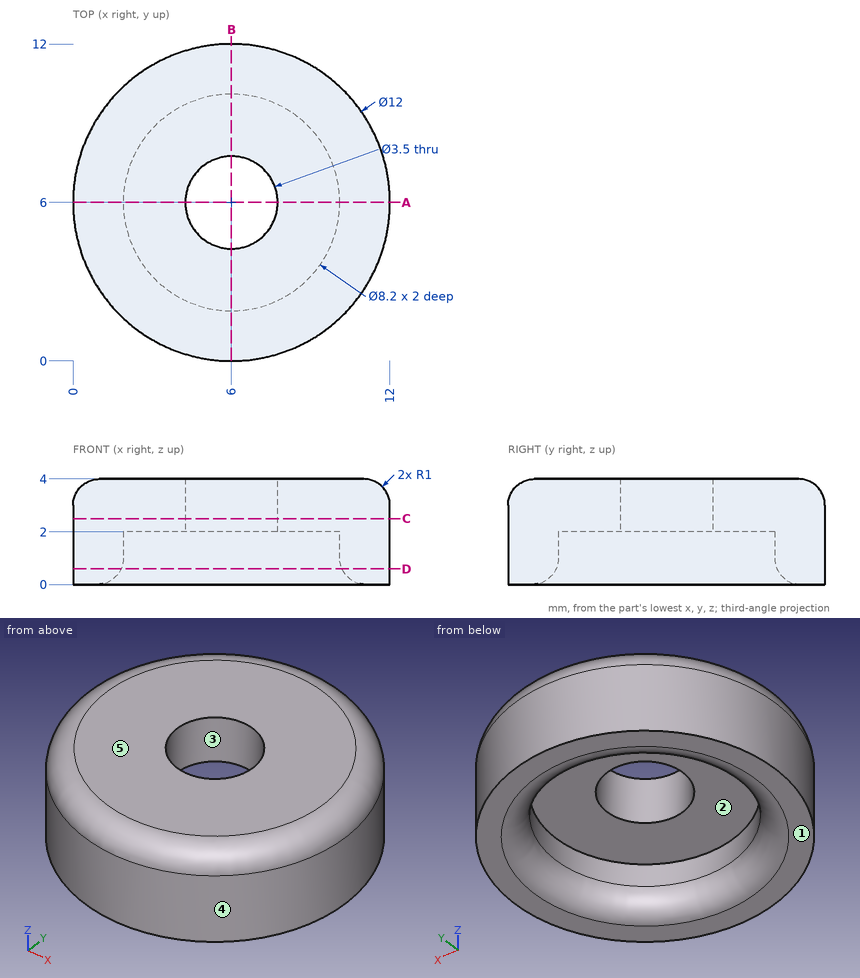
Geometry check sheet. Reference: drawing and pictorial views, mm from the part's lowest x, y, z. A direction names the side the tool comes from. Round coordinates to 2 decimals unless told otherwise and drop trailing zeros. Write each loop counter-clockwise with the first axis right and the second up, starting at its lowest first coordinate (ties: lowest second). Pieces come first, ordered by that corner, then holes. Notation, with made-up numbers: (2, 11) -> (19, 11) arc R21 ccw to (19, 43) -> close; hole circle Ø9 at (27.25, 84). An arc over 180 degrees is marked (long way). Put each result on its own line as item: value.
1) Access from +Z, -Z, +X, -X, +Y, -Y to the whole of each face (thin tool, end or side, straight path). Record for the marked faces 1 and 2.
Recorded:
face 1: -Z, +X, -X, +Y, -Y
face 2: -Z
2) Cross-section at A-A, the plane y = 6. Enter the section's corners in (x, z), plus the area to 3 significant figures.
Recorded:
outline: (0, 0) -> (0.9, 0) arc R1 ccw to (1.9, 1) -> (1.9, 2) -> (4.25, 2) -> (4.25, 4) -> (1, 4) arc R1 ccw to (0, 3) -> close; (7.75, 2) -> (10.1, 2) -> (10.1, 1) arc R1 ccw to (11.1, 0) -> (12, 0) -> (12, 3) arc R1 ccw to (11, 4) -> (7.75, 4) -> close
area: 23.7 mm2
3) Cross-section at C-C, the plane z = 2.5. Enter the section's corners in (x, y).
Recorded:
outline: circle Ø12 at (6, 6); hole circle Ø3.5 at (6, 6)
4) Cross-section at D-D, the plane z = 0.6. Enter the section's corners in (x, y).
Recorded:
outline: circle Ø12 at (6, 6); hole circle Ø8.37 at (6, 6)
5) Release check for a two-part mould opening along Y. For the marked faces 3, 4 and 5 record: pulls with the +Y half, pulls with the -Y half, needs draft (parallel to the pull), parting line crosses it, or undercut.
Recorded:
face 3: undercut
face 4: parting line crosses it
face 5: needs draft
6) Thickness scan on probe 1 along Y at (x, z) = (6, 1.7); probe 2 along Z at (x, y) = (8.25, 5); probe 3 along Y at (x, z) = (5.25, 2.1). Record the ranges inside material, lowest first. Write a range as from..to.
Recorded:
probe 1: y = 0..1.9, 10.1..12
probe 2: z = 2..4
probe 3: y = 0.05..4.42, 7.58..11.95
7) Depth check by flat-ended pin: P1, Ø4, axis at x = 6, y = 6, coming from the -Z side; P2, Ø2, axis at x = 7, z = 0.5, coming from the +Y side; P3, Ø1.5, axis at y = 7, z = 1.5, coming from the -X side; P4, Ø1.5, axis at y = 10.5, z = 2, coming from the -X side. Enter the tip coordinate at first touch or a pass-through.
Recorded:
P1: stops at z = 2
P2: stops at y = 12
P3: stops at x = 0.01
P4: stops at x = 1.32
